Geometry: see drawing. Coordinates: mm, zero at the bounding-box minimum. Give positions to 0.01 mm unless a question says otherwise; leave off trailing zeros. Write each loop counter-clockwise with the first axis right and the second up, starting at its lowest first coordinate (ties: lowest second). Pieces come first, ordered by that corner, then holes. Notation, with made-up numbers: M 39,39.25 L 48,39.25 A21 cw 48,47.25 Z; hole C -8,46 d7. An arc over 180 degrees is marked long. Use one line per item in the form item = value. Start each with the question number.
Item 1: Section query C-C on y = 2.2. Give the number of separate pieces and of enclosed holes in the cut face, then the cut area to 3 significant figures.
Item 2: Section query A-A on z = 48. Return loops of the section in (x, y), then the cut area to 3 significant figures.
Item 3: Contact query for a flat-ended pin moving along its axis: P1, Ø3, axis at x = 167.8, z = 10, coming from the +Y side. Output: stop coordinate, or through.
Item 4: Section query D-D on z = 61.5. Return loops of the section in (x, y), then the cut area to 3 significant figures.
Item 5: Section query B-B on x = 20. Return loops of the section in (y, z).
Item 6: Material intervals for line 1 along X through (y, z) = (1.2, 70.5); line 2 along X through (y, z) = (1.7, 69); line 3 along X through (y, z) = (0.9, 30.5), sorted ascending. Write a range as from..to.
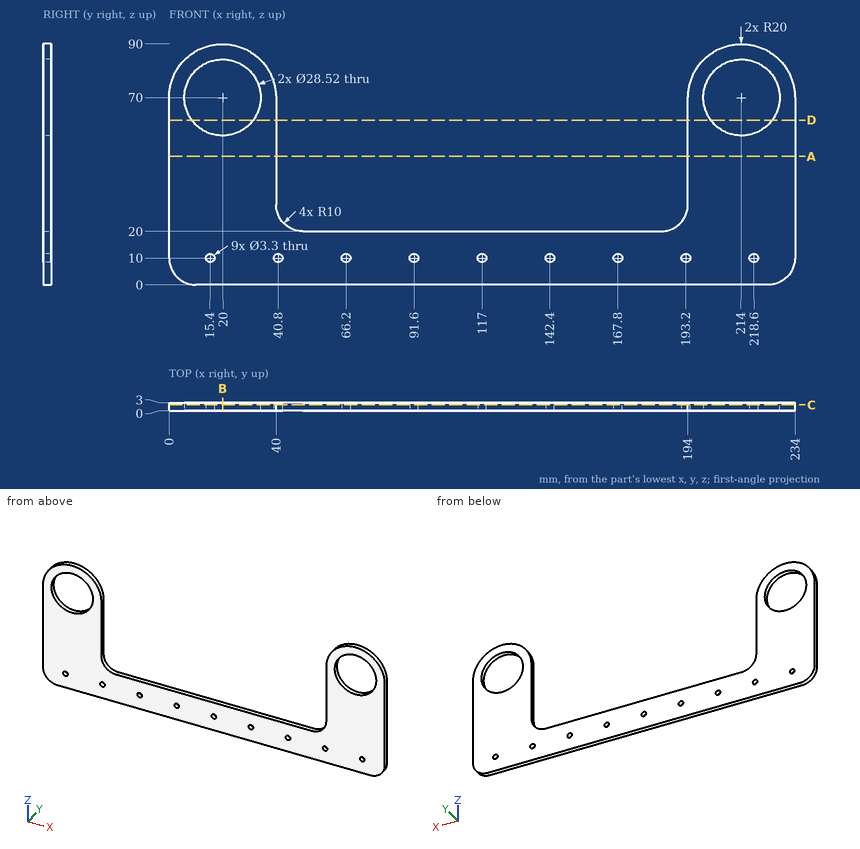
Answer sheet:
q1.separate_pieces = 1
q1.enclosed_holes = 11
q1.area = 8,580 mm2
q2.outline = M 0,0 L 40,0 L 40,3 L 0,3 Z; M 194,0 L 234,0 L 234,3 L 194,3 Z
q2.area = 240 mm2
q3.P1 = through
q4.outline = M 0,0 L 8.55,0 L 8.55,3 L 0,3 Z; M 31.45,0 L 40,0 L 40,3 L 31.45,3 Z; M 194,0 L 202.55,0 L 202.55,3 L 194,3 Z; M 225.45,0 L 234,0 L 234,3 L 225.45,3 Z
q4.area = 103 mm2
q5.outline = M 0,0 L 3,0 L 3,55.74 L 0,55.74 Z; M 0,84.26 L 3,84.26 L 3,90 L 0,90 Z
q6.line_1 = 0.01..5.75, 34.25..39.99, 194.01..199.75, 228.25..233.99
q6.line_2 = 0..5.78, 34.22..40, 194..199.78, 228.22..234
q6.line_3 = 0..40, 194..234
